```python
from build123d import *

# Parameters (mm, degrees)
BOSS_EXTRUDE1_DEPTH = 95.25
CUT_EXTRUDE1_DEPTH  = 95.25


with BuildPart() as part:
    # Sketch2 → Boss-Extrude1 (new body)
    with BuildSketch(Plane.XY):
        with BuildLine():
            Line((38.1, 1.3208), (82.55, 1.3208))
            Line((82.55, 1.3208), (82.55, -1.3208))
            Line((82.55, -1.3208), (-82.55, -1.3208))
            Line((-82.55, -1.3208), (-82.55, 1.3208))
            Line((-82.55, 1.3208), (-38.1, 1.3208))
            Line((-38.1, 1.3208), (-38.1, 27.074795193))
            ThreePointArc((-38.1, 27.074795193), (0, 16.0782), (38.1, 27.074795193))
            Line((38.1, 27.074795193), (38.1, 1.3208))
        make_face()
    extrude(amount=BOSS_EXTRUDE1_DEPTH)

    # Sketch3 → Cut-Extrude1 (cut)
    with BuildSketch(Plane(origin=(0, 1.3208, 0), x_dir=(1, 0, 0), z_dir=(0, 1, 0))):
        with BuildLine():
            Line((-77.47, -5.207), (-46.482, -5.207))
            ThreePointArc((-46.482, -5.207), (-42.164, -9.525), (-46.482, -13.843))
            Line((-46.482, -13.843), (-77.47, -13.843))
            ThreePointArc((-77.47, -13.843), (-81.788, -9.525), (-77.47, -5.207))
        make_face()
        with BuildLine():
            Line((-77.47, -81.407), (-46.482, -81.407))
            ThreePointArc((-46.482, -81.407), (-42.164, -85.725), (-46.482, -90.043))
            Line((-46.482, -90.043), (-77.47, -90.043))
            ThreePointArc((-77.47, -90.043), (-81.788, -85.725), (-77.47, -81.407))
        make_face()
    cut_extrude1 = extrude(amount=-CUT_EXTRUDE1_DEPTH, mode=Mode.SUBTRACT)

    # Mirror2: Cut-Extrude1 across plane
    add(cut_extrude1.mirror(Plane(origin=(0, 0, 0), x_dir=(0, 0, 1), z_dir=(1, 0, 0))), mode=Mode.SUBTRACT)


solid = part.part
```
Geometry check sheet. Reference: the model listing, model coordinates, mm. A direction names the side the tool comes from. Coordinates: 2 decimals unless noted, no trailing zeros. Loops run counter-clockwise (first coordinate to the right, second up) from the corner with the lowest first, then second, coordinate; pieces in that order, holes last.
Item 1: Release check for a two-part mould opening along Z. For faces 6 (the face through (42.165, 0.018, 9.43)), 7 (the face through (1, -1.321, 47)), 8 (the face through (1, 10, 0)) record: released by +Z, released by -Z, zero draft, split by the parting line, or undercut.
Item 2: Access from +Z, -Z, +X, -X, +Y, -Y to the whole of each face (thin tool, end or side, straight path). Record for faces 1 (the face through (81.787, 0.018, 9.62)), 2 (the face through (1, 10, 95.25)), 3 (the face through (-0.56, 16.08, 46.96)), 4 (the face through (38.1, 14, 47)), 5 (the face through (-61, 1.321, 47)).
Item 3: Sectioned sample at B-B, the plane z = 48. Record the boundary of the cut face in (x, y).
Item 4: Sectioned sample at D-D, the plane y = 12. Record the boundary of the cut face in (x, z).
Item 5: Sectioned sample at A-A, the plane x = -67. Record the boundary of the cut face in (y, z), then the cut area to 3 significant figures.
Item 6: Go/stop test with flat-tipped pins: pin 1 Ø7.5 at (y, z) = (16.5, 51) entering from -X; pin 2 Ø8 at (x, z) = (14, 18.5) entering from +Y; pin 3 Ø6 at (y, z) = (9.5, 67.5) entering from +X. Record where each tip stops, or that it passes through.
Item 7: Sectioned sample at C-C, the plane y = 19. Record the boundary of the cut face in (x, z).
Item 8: Thickness scan on line 1 (Y direction, x = -2, z = 84); line 2 (X direction, y = 5.25, z = 39.5); line 3 (Y direction, x = -70, z = 14). Record the ranges inside material, lowest first.
Check result:
1. face 6: undercut
1. face 7: zero draft
1. face 8: released by -Z
2. face 1: +Y, -Y
2. face 2: +Z, +X, -X, +Y, -Y
2. face 3: +Z, -Z, +Y
2. face 4: +Z, -Z, +X, +Y
2. face 5: +Z, -Z, -X, +Y
3. outline: (-82.55, -1.32) - (82.55, -1.32) - (82.55, 1.32) - (38.1, 1.32) - (38.1, 27.07) arc R71.5 cw to (-38.1, 27.07) - (-38.1, 1.32) - (-82.55, 1.32) - close
4. outline: (-38.1, 0) - (38.1, 0) - (38.1, 95.25) - (-38.1, 95.25) - close
5. outline: (-1.32, 0) - (1.32, 0) - (1.32, 5.21) - (-1.32, 5.21) - close; (-1.32, 13.84) - (1.32, 13.84) - (1.32, 81.41) - (-1.32, 81.41) - close; (-1.32, 90.04) - (1.32, 90.04) - (1.32, 95.25) - (-1.32, 95.25) - close
5. area: 206 mm2
6. pin 1: stops at x = -38.1
6. pin 2: stops at y = 18.38
6. pin 3: stops at x = 38.1
7. outline: (-38.1, 0) - (-20.23, 0) - (-20.23, 95.25) - (-38.1, 95.25) - close; (20.23, 0) - (38.1, 0) - (38.1, 95.25) - (20.23, 95.25) - close
8. line 1: y = -1.32 to 16.11
8. line 2: x = -38.1 to 38.1
8. line 3: y = -1.32 to 1.32
